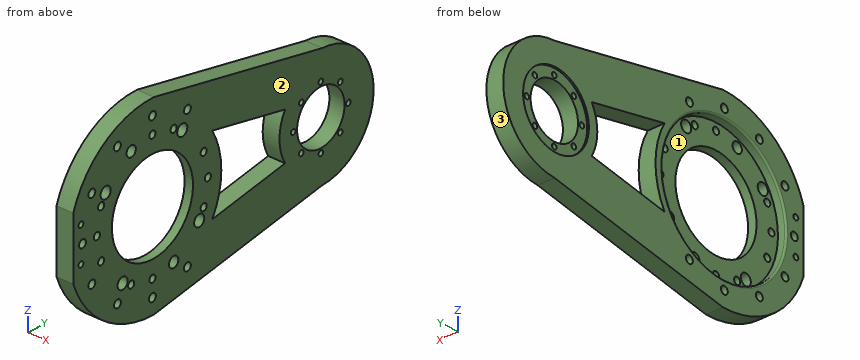
```python
from build123d import *

# Parameters (mm, degrees)
SKETCH2_R                       = 40.5
SKETCH2_R_2                     = 15.5
BOSS_EXTRUDE1_DEPTH             = 5
BOSS_EXTRUDE2_START             = -5
SKETCH2_5_R                     = 40.5
SKETCH2_5_R_2                   = 15.5
BOSS_EXTRUDE2_DEPTH             = 5
FILLET3_R                       = 1
SKETCH12_R                      = 1.5
CUT_EXTRUDE12_DEPTH             = 191.422110061
CIRPATTERN1_COUNT               = 8
SKETCH13_R                      = 21.5
CUT_EXTRUDE13_DEPTH             = 1
CUT_EXTRUDE16_DEPTH             = 10
SKETCH16_W                      = 105.253324721
SKETCH16_H                      = 10.065806818
CUT_EXTRUDE17_DEPTH             = 10
CUT_EXTRUDE20_DEPTH             = 155.830035846
SKETCH29_R                      = 1.6
CUT_EXTRUDE21_DEPTH             = 10
SKETCH31_R                      = 2.25
CUT_EXTRUDE22_DEPTH             = 10
CIRPATTERN2_COUNT               = 5
CIRPATTERN2_ANGLE               = 120
CIRPATTERN2_THE_OTHER_WAY_COUNT = 5
CIRPATTERN2_THE_OTHER_WAY_ANGLE = 120


with BuildPart() as part:
    # Sketch2 → Boss-Extrude1 (new body)
    # profile 1 of 2: a face of its own
    with BuildSketch(Plane(origin=(0, 0, 0), x_dir=(0, 0, -1), z_dir=(1, 0, 0))):
        with BuildLine():
            Line((-67.7, 110), (-67.7, 0))
            Line((-67.7, 0), (-67.7, -68))
            Line((-67.7, -68), (67.7, -68))
            Line((67.7, -68), (67.7, 10))
            Line((67.7, 10), (67.7, 110))
            ThreePointArc((67.7, 110), (0, 177.7), (-67.7, 110))
        make_face()
        Circle(SKETCH2_R, mode=Mode.SUBTRACT)
        with Locations((0, 110)):
            Circle(SKETCH2_R_2, mode=Mode.SUBTRACT)
    # profile 2 of 2: a face of its own
    with BuildSketch(Plane(origin=(0, 0, 0), x_dir=(0, 0, -1), z_dir=(1, 0, 0))):
        Circle(SKETCH2_R)
        with BuildLine():
            ThreePointArc((-17.143658425, -32.906392289), (-21.81056318, -32.906392289), (-21.81056318, -28.239487533))
            ThreePointArc((-21.81056318, -28.239487533), (-17.143658425, -28.239487533), (-17.143658425, -32.906392289))
        make_face(mode=Mode.SUBTRACT)
        with BuildLine():
            ThreePointArc((-35.647308736, -11.715598741), (-31.333957371, -11.715598741), (-31.333957371, -16.028950106))
            ThreePointArc((-31.333957371, -16.028950106), (-35.647308736, -16.028950106), (-35.647308736, -11.715598741))
        make_face(mode=Mode.SUBTRACT)
        with BuildLine():
            ThreePointArc((-12.458060861, -34.904846616), (-15.286487986, -34.904846616), (-15.286487986, -32.076419491))
            ThreePointArc((-15.286487986, -32.076419491), (-12.458060861, -32.076419491), (-12.458060861, -34.904846616))
        make_face(mode=Mode.SUBTRACT)
        with BuildLine():
            ThreePointArc((-37.664213562, 1.414213562), (-34.835786438, 1.414213562), (-34.835786438, -1.414213562))
            ThreePointArc((-34.835786438, -1.414213562), (-37.664213562, -1.414213562), (-37.664213562, 1.414213562))
        make_face(mode=Mode.SUBTRACT)
        with BuildLine():
            ThreePointArc((-32.076419491, 12.458060861), (-34.904846616, 12.458060861), (-34.904846616, 15.286487986))
            ThreePointArc((-34.904846616, 15.286487986), (-32.076419491, 15.286487986), (-32.076419491, 12.458060861))
        make_face(mode=Mode.SUBTRACT)
        with BuildLine():
            ThreePointArc((-28.239487533, 17.143658425), (-32.906392289, 17.143658425), (-32.906392289, 21.81056318))
            ThreePointArc((-32.906392289, 21.81056318), (-28.239487533, 21.81056318), (-28.239487533, 17.143658425))
        make_face(mode=Mode.SUBTRACT)
        with BuildLine():
            ThreePointArc((-15.286487986, 34.904846616), (-12.458060861, 34.904846616), (-12.458060861, 32.076419491))
            ThreePointArc((-12.458060861, 32.076419491), (-15.286487986, 32.076419491), (-15.286487986, 34.904846616))
        make_face(mode=Mode.SUBTRACT)
        with BuildLine():
            ThreePointArc((-1.414213562, 37.664213562), (1.414213562, 37.664213562), (1.414213562, 34.835786438))
            ThreePointArc((1.414213562, 34.835786438), (-1.414213562, 34.835786438), (-1.414213562, 37.664213562))
        make_face(mode=Mode.SUBTRACT)
        with BuildLine():
            ThreePointArc((-1.414213562, -34.835786438), (1.414213562, -34.835786438), (1.414213562, -37.664213562))
            ThreePointArc((1.414213562, -37.664213562), (-1.414213562, -37.664213562), (-1.414213562, -34.835786438))
        make_face(mode=Mode.SUBTRACT)
        with BuildLine():
            ThreePointArc((12.458060861, -32.076419491), (15.286487986, -32.076419491), (15.286487986, -34.904846616))
            ThreePointArc((15.286487986, -34.904846616), (12.458060861, -34.904846616), (12.458060861, -32.076419491))
        make_face(mode=Mode.SUBTRACT)
        with BuildLine():
            ThreePointArc((32.906392289, -21.81056318), (28.239487533, -21.81056318), (28.239487533, -17.143658425))
            ThreePointArc((28.239487533, -17.143658425), (32.906392289, -17.143658425), (32.906392289, -21.81056318))
        make_face(mode=Mode.SUBTRACT)
        with BuildLine():
            ThreePointArc((34.904846616, -15.286487986), (32.076419491, -15.286487986), (32.076419491, -12.458060861))
            ThreePointArc((32.076419491, -12.458060861), (34.904846616, -12.458060861), (34.904846616, -15.286487986))
        make_face(mode=Mode.SUBTRACT)
        with BuildLine():
            ThreePointArc((16.292073099, 20.900199859), (20.900199859, -16.292073099), (-16.292073099, -20.900199859))
            ThreePointArc((-16.292073099, -20.900199859), (-20.900199859, 16.292073099), (16.292073099, 20.900199859))
        make_face(mode=Mode.SUBTRACT)
        with BuildLine():
            ThreePointArc((35.647308736, 11.715598741), (31.333957371, 11.715598741), (31.333957371, 16.028950106))
            ThreePointArc((31.333957371, 16.028950106), (35.647308736, 16.028950106), (35.647308736, 11.715598741))
        make_face(mode=Mode.SUBTRACT)
        with BuildLine():
            ThreePointArc((12.458060861, 34.904846616), (15.286487986, 34.904846616), (15.286487986, 32.076419491))
            ThreePointArc((15.286487986, 32.076419491), (12.458060861, 32.076419491), (12.458060861, 34.904846616))
        make_face(mode=Mode.SUBTRACT)
        with BuildLine():
            ThreePointArc((21.81056318, 28.239487533), (17.143658425, 28.239487533), (17.143658425, 32.906392289))
            ThreePointArc((17.143658425, 32.906392289), (21.81056318, 32.906392289), (21.81056318, 28.239487533))
        make_face(mode=Mode.SUBTRACT)
        with BuildLine():
            ThreePointArc((34.835786438, 1.414213562), (37.664213562, 1.414213562), (37.664213562, -1.414213562))
            ThreePointArc((37.664213562, -1.414213562), (34.835786438, -1.414213562), (34.835786438, 1.414213562))
        make_face(mode=Mode.SUBTRACT)
    extrude(amount=BOSS_EXTRUDE1_DEPTH)

    # Sketch2<5> → Boss-Extrude2 (add)
    with BuildSketch(Plane(origin=(0, 0, 0), x_dir=(0, 0, -1), z_dir=(1, 0, 0)).offset(BOSS_EXTRUDE2_START)):
        with BuildLine():
            Line((-67.7, 110), (-67.7, 0))
            Line((-67.7, 0), (-67.7, -68))
            Line((-67.7, -68), (67.7, -68))
            Line((67.7, -68), (67.7, 10))
            Line((67.7, 10), (67.7, 110))
            ThreePointArc((67.7, 110), (0, 177.7), (-67.7, 110))
        make_face()
        Circle(SKETCH2_5_R, mode=Mode.SUBTRACT)
        with Locations((0, 110)):
            Circle(SKETCH2_5_R_2, mode=Mode.SUBTRACT)
    extrude(amount=BOSS_EXTRUDE2_DEPTH)

    # Fillet3
    fillet3_edges = [part.edges().sort_by_distance(p)[0] for p in [
        (-5, 0, 40.5),
    ]]
    fillet(fillet3_edges, radius=FILLET3_R)

    # Sketch12 → Cut-Extrude12 (cut, through all)
    with BuildSketch(Plane.ZY.offset(5)):
        with Locations((-0.00151734, 127.999999936)):
            Circle(SKETCH12_R)
    cut_extrude12 = extrude(amount=-CUT_EXTRUDE12_DEPTH, mode=Mode.SUBTRACT)

    # CirPattern1: Cut-Extrude12 ×8 about axis
    cirpattern1_axis = Axis((0, 110, 0), (1, 0, 0))
    for i in range(1, CIRPATTERN1_COUNT):
        add(cut_extrude12.rotate(cirpattern1_axis, i * 360 / CIRPATTERN1_COUNT), mode=Mode.SUBTRACT)

    # Sketch13 → Cut-Extrude13 (cut)
    with BuildSketch(Plane.ZY.offset(5)):
        with Locations((0, 110)):
            Circle(SKETCH13_R)
    extrude(amount=-CUT_EXTRUDE13_DEPTH, mode=Mode.SUBTRACT)

    # Sketch15 → Cut-Extrude16 (cut)
    with BuildSketch(Plane.ZY.offset(5)):
        with BuildLine():
            ThreePointArc((67.7, 110), (0, 177.7), (-67.7, 110))
            Line((-67.7, 110), (-67.7, -68))
            Line((-67.7, -68), (67.7, -68))
            Line((67.7, -68), (67.7, 110))
        make_face()
        with BuildLine():
            ThreePointArc((-54.691644033, 0.956071637), (0, -54.7), (54.691644033, 0.956071637))
            Line((54.691644033, 0.956071637), (34.485862883, 110.987553146))
            ThreePointArc((34.485862883, 110.987553146), (0, 144.5), (-34.485862883, 110.987553146))
            Line((-34.485862883, 110.987553146), (-54.691644033, 0.956071637))
        make_face(mode=Mode.SUBTRACT)
    extrude(amount=-CUT_EXTRUDE16_DEPTH, mode=Mode.SUBTRACT)

    # Sketch16 → Cut-Extrude17 (cut)
    with BuildSketch(Plane.ZY.offset(5)):
        with Locations((1.105505895, -56.732903409)):
            Rectangle(SKETCH16_W, SKETCH16_H)
    extrude(amount=-CUT_EXTRUDE17_DEPTH, mode=Mode.SUBTRACT)

    # Sketch19 → Cut-Extrude20 (cut, through all)
    with BuildSketch(Plane(origin=(5, 0, 0), x_dir=(0, 0, -1), z_dir=(1, 0, 0))):
        with BuildLine():
            ThreePointArc((22.268259026, 39.104023322), (0, 45), (-22.268259026, 39.104023322))
            Line((-22.268259026, 39.104023322), (-13.538953214, 86.63984705))
            ThreePointArc((-13.538953214, 86.63984705), (0, 83), (13.538953214, 86.63984705))
            Line((13.538953214, 86.63984705), (22.268259026, 39.104023322))
        make_face()
    extrude(amount=-CUT_EXTRUDE20_DEPTH, mode=Mode.SUBTRACT)

    # Sketch29 → Cut-Extrude21 (cut)
    with BuildSketch(Plane(origin=(5, 0, 0), x_dir=(0, 0, -1), z_dir=(1, 0, 0))):
        with Locations((-10, -46.7)):
            Circle(SKETCH29_R)
        with Locations((10, -46.7)):
            Circle(SKETCH29_R)
    extrude(amount=-CUT_EXTRUDE21_DEPTH, mode=Mode.SUBTRACT)

    # Sketch31 → Cut-Extrude22 (cut)
    with BuildSketch(Plane(origin=(5, 0, 0), x_dir=(0, 0, -1), z_dir=(1, 0, 0))):
        with Locations((0, -45.7)):
            Circle(SKETCH31_R)
    cut_extrude22 = extrude(amount=-CUT_EXTRUDE22_DEPTH, mode=Mode.SUBTRACT)

    # CirPattern2: Cut-Extrude22 ×5 about axis
    cirpattern2_axis = Axis((0, 0, 0), (-1, 0, 0))
    for i in range(1, CIRPATTERN2_COUNT):
        add(cut_extrude22.rotate(cirpattern2_axis, i * CIRPATTERN2_ANGLE / (CIRPATTERN2_COUNT - 1)), mode=Mode.SUBTRACT)

    # CirPattern2 the other way: Cut-Extrude22 ×5 about axis
    cirpattern2_the_other_way_axis = Axis((0, 0, 0), (1, 0, 0))
    for i in range(1, CIRPATTERN2_THE_OTHER_WAY_COUNT):
        add(cut_extrude22.rotate(cirpattern2_the_other_way_axis, i * CIRPATTERN2_THE_OTHER_WAY_ANGLE / (CIRPATTERN2_THE_OTHER_WAY_COUNT - 1)), mode=Mode.SUBTRACT)


solid = part.part
```
Geometry: final body of the model. Coordinates: model frame, mm. Face numbers are marked on the shaded views. Give positions to 0.01 mm unless a question says otherwise; leave off trailing zeros. Write each loop counter-clockwise with the first axis right and the second up, starting at its lowest first coordinate (ties: lowest second). Pieces come first, ordered by that corner, then holes.
1. Section query A-A, the plane y = 116. Return loops of the section in (x, z), then the cut area to 3 significant figures.
2. Line query: probe 1 along Z at (x, y) = (0.5, 0); probe 2 along Z at (x, y) = (2.5, 109); probe 3 along Y at (x, z) = (-1.5, -23). Output: solid intervals per line, ascending.
3. Draft query along Y for the marked faces 1, 2 and 3. Return one class per face: released by +Y, released by -Y, zero draft, split by the parting line, or undercut.
4. Section query B-B, the plane x = -2.5. Count the separate pieces of the cut face and the enclosed holes in it, then the cut area to 4 significant figures.
5. Pin query (flat end, axial travel): P1, Ø6, axis at x = 0.5, y = 116, coming from the +Z side; P2, Ø1.5, axis at x = -1.5, y = -29, coming from the -Z side; P3, Ø5, axis at y = 33.49, z = -13.87, coming from the -X side. Return the tip coordinate at first contact, or that it passes through.
Computed:
1. outline: (-5, -33.97) - (5, -33.97) - (5, -14.29) - (-4, -14.29) - (-4, -20.65) - (-5, -20.65) - close; (-5, 20.65) - (-4, 20.65) - (-4, 14.29) - (5, 14.29) - (5, 33.97) - (-5, 33.97) - close
1. area: 381 mm2
2. probe 1: z = -54.7 to -47.95, -43.45 to -38.25, -34.25 to -26.5, 26.5 to 34.25, 38.25 to 43.45, 47.95 to 54.7
2. probe 2: z = -34.85 to -19.12, -16.88 to -15.47, 15.47 to 16.88, 19.12 to 34.85
2. probe 3: y = -49.63 to -41.82, -37.33 to -33.34, 33.34 to 135.71
3. face 1: undercut
3. face 2: zero draft
3. face 3: released by +Y
4. separate pieces: 1
4. enclosed holes: 22
4. area: 8,765 mm2
5. P1: stops at z = 34.37
5. P2: stops at z = -46.84
5. P3: stops at x = 0
